Can you work these out from the model? Positions are in its coordinate system, mm. A direction names the side the tool comes from. Give positions to 0.01 mm unless a question says otherwise; leave off trailing zeros. Loops run counter-clockwise (first coordinate to the right, second up) from the corner with the lowest first, then second, coordinate; pieces in that order, holes last.
from build123d import *

# Parameters (mm, degrees)
PAD002_DEPTH    = 4.1
SKETCH017_W     = 2.7
SKETCH017_H     = 13
POCKET011_DEPTH = 10.7735
SKETCH018_W     = 1.55
SKETCH018_H     = 2
POCKET012_DEPTH = 27.001
SKETCH019_R     = 1.24
PAD003_DEPTH    = 2.2
CHAMFER001_SIZE = 0.4


with BuildPart() as body003:
    # Sketch016 (on DatumPlane) → Pad002 (new body, symmetric)
    with BuildSketch(Plane.YZ.offset(1.27)):
        with BuildLine():
            Line((0.91, 7.4), (3.71, 7.4))
            Line((3.71, 7.4), (3.71, 21.95))
            Line((3.71, 21.95), (3.01, 21.95))
            Line((3.01, 21.95), (3.01, 21.45))
            Line((1.71, 21.45), (3.01, 21.45))
            Line((1.71, 21.45), (1.71, 23.2))
            Line((1.71, 23.2), (5.36, 27))
            Line((7.61, 27), (5.36, 27))
            Line((7.61, 27), (7.564167, 22))
            Line((7.564167, 22), (8.71, 17))
            Line((8.71, 17), (10.7725, 8))
            Line((10.7725, 8), (5.86, 5.2))
            Line((5.86, 5.2), (3.11, 5.2))
            ThreePointArc((0.91, 7.4), (1.554365, 5.844365), (3.11, 5.2))
        make_face()
    extrude(amount=PAD002_DEPTH, both=True)

    # Sketch017 → Pocket011 (cut, through all)
    with BuildSketch(Plane.XZ):
        with Locations((4.02, 11)):
            Rectangle(SKETCH017_W, SKETCH017_H)
        with Locations((-1.48, 11)):
            Rectangle(SKETCH017_W, SKETCH017_H)
    extrude(amount=-POCKET011_DEPTH, mode=Mode.SUBTRACT)

    # Sketch018 → Pocket012 (cut, through all)
    with BuildSketch(Plane.XY):
        with Locations((-2.055, 2.71)):
            Rectangle(SKETCH018_W, SKETCH018_H)
        with Locations((4.595, 2.71)):
            Rectangle(SKETCH018_W, SKETCH018_H)
    extrude(amount=POCKET012_DEPTH, mode=Mode.SUBTRACT)

    # Sketch019 (on DatumPlane) → Pad003 (join, symmetric)
    with BuildSketch(Plane.YZ.offset(1.27)):
        with Locations((5.86, 9.54)):
            Circle(SKETCH019_R)
    extrude(amount=PAD003_DEPTH, both=True)

    # Chamfer001
    chamfer001_edges = [body003.edges().sort_by_distance(p)[0] for p in [
        (1.27, 1.71, 21.45),
        (1.27, 3.01, 21.45),
    ]]
    chamfer(chamfer001_edges, length=CHAMFER001_SIZE)


with BuildPart() as part_mirroring:
    # Part__Mirroring: instance of Body003
    add(body003.part.mirror(Plane(origin=(0, -8.89, 0), x_dir=(1, 0, 0), z_dir=(0, 1, 0))))


solid = part_mirroring.part
(1) Which directions (+Z, -Z, +X, -X, +Y, -Y) give clear straight access to the entire face, cutting with the end or side of a thin tool? Please do faces 1 (the flat face through (3.47, -24, 10)), 2 (the cylindrical face through (-0.52, -23.37, 8.33)), 3 (the cylindrical face through (3.08, -23.37, 8.33)), 4 (the flat face through (3.82, -21, 23)), 5 (the flat face through (-1, -24, 17.5)).
Returned:
face 1: -Z, +X, +Y, -Y
face 2: -X
face 3: +X
face 4: +Z, -Z, +X, +Y
face 5: -X, +Y, -Y
(2) Suppose I cut it at D-D on z = 23.5. List the corners of the cut face in (x, y) for me.
Returned:
outline: (-2.83, -25.36) - (5.37, -25.36) - (5.37, -21.49) - (3.82, -21.49) - (3.82, -19.78) - (-1.28, -19.78) - (-1.28, -21.49) - (-2.83, -21.49) - close
(3) Suppose I cut it at B-B on x = 1. List the corners of the cut face in (y, z) for me, plus the area to 3 significant figures.
Returned:
outline: (-28.55, 8) - (-23.64, 5.2) - (-20.89, 5.2) arc R2.2 ccw to (-18.69, 7.4) - (-21.49, 7.4) - (-21.49, 21.95) - (-20.79, 21.95) - (-20.79, 21.85) - (-20.39, 21.45) - (-19.89, 21.45) - (-19.49, 21.85) - (-19.49, 23.2) - (-23.14, 27) - (-25.39, 27) - (-25.34, 22) - close
area: 117 mm2
(4) Please list where these lines run through material, in increasing order: probe 1 along X at (y, z) = (-24, 15.25); probe 2 along Z at (x, y) = (4, -24.5); probe 3 along X at (y, z) = (-23.75, 9).
Returned:
probe 1: x = -0.13 to 2.67
probe 2: z = 17.5 to 27
probe 3: x = -0.93 to 3.47
(5) Will these pins go through, and if not, where does the flat tip stop? P1, Ø1.3, axis at x = 4.5, y = -25, coming from the -Z side; P2, Ø2.5, axis at y = -23.5, z = 9.5, coming from the +X side; P3, Ø2, axis at x = 1, y = -20, coming from the -Z side; P4, Ø1, axis at x = 3, y = -24.5, coming from the -Z side.
Returned:
P1: stops at z = 17.5
P2: stops at x = 3.47
P3: stops at z = 5.2
P4: stops at z = 5.48
(6) Suppose I cut it at C-C on y = -22.75. List the corners of the cut face in (x, z) for me, plus the area to 3 significant figures.
Returned:
outline: (-2.83, 17.5) - (-0.13, 17.5) - (-0.13, 10.4) - (-0.93, 10.4) - (-0.93, 8.68) - (-0.13, 8.68) - (-0.13, 5.2) - (2.67, 5.2) - (2.67, 8.68) - (3.47, 8.68) - (3.47, 10.4) - (2.67, 10.4) - (2.67, 17.5) - (5.37, 17.5) - (5.37, 26.59) - (-2.83, 26.59) - close
area: 112 mm2
(7) Suppose I cut it at A-A on x = 3.25. List the corners of the cut face in (y, z) for me.
Returned:
outline: (-26.38, 17.5) - (-21.49, 17.5) - (-21.49, 21.95) - (-20.79, 21.95) - (-20.79, 21.85) - (-20.39, 21.45) - (-19.89, 21.45) - (-19.49, 21.85) - (-19.49, 23.2) - (-23.14, 27) - (-25.39, 27) - (-25.34, 22) - close; circle Ø2.48 at (-23.64, 9.54)
